```python
from build123d import *

# Parameters (mm, degrees)
F0_W     = 50.8
F0_H     = 33.02
F0_W_2   = 40.64
F0_H_2   = 22.86
F1_DEPTH = 17.78
F2_DEPTH = 12.7
F3_R     = 3.175
F4_DEPTH = 254


with BuildPart() as f1:
    # F0 (on Top) → F1 (new body)
    with BuildSketch(Plane.XY):
        with Locations((-7.5921734202, -29.6402639918)):
            Rectangle(F0_W, F0_H)
        with Locations((-7.5921734202, -29.6402639918)):
            Rectangle(F0_W_2, F0_H_2, mode=Mode.SUBTRACT)
        with Locations((-7.5921734202, -29.6402639918)):
            Rectangle(F0_W_2, F0_H_2)
    extrude(amount=F1_DEPTH)

    # F0 (on Top) → F2 (cut)
    with BuildSketch(Plane.XY):
        with Locations((-7.5921734202, -29.6402639918)):
            Rectangle(F0_W_2, F0_H_2)
    extrude(amount=F2_DEPTH, mode=Mode.SUBTRACT)

    # F3 (on face) → F4 (cut)
    with BuildSketch(Plane(origin=(-32.9921734202, 0, 0), x_dir=(0, -1, 0), z_dir=(-1, 0, 0))):
        with Locations((29.6402639918, 9.4274014091)):
            Circle(F3_R)
    extrude(amount=-F4_DEPTH, mode=Mode.SUBTRACT)


solid = f1.part
```
Can you work these out from the model? Positions are in its coordinate system, mm. A direction names the side the tool comes from. Coordinates: 2 decimals unless noted, no trailing zeros. Loops run counter-clockwise (first coordinate to the right, second up) from the corner with the lowest first, then second, coordinate; pieces in that order, holes last. Notation, with made-up numbers: (-23, -16) -> (-9, -16) arc R23 ccw to (-9, -6) -> close; hole circle Ø4 at (13, 75). An arc over 180 degrees is marked (long way). Answer as a JSON object with one key per item and string values.
1) Thinking about a two-plate mould opening in Y: for faces 1 (the face through (-27.912, -30, 5)), 2 (the face through (17.808, -26, 9)), 3 (the face through (-30.488, -32.573, 8.211)), 4 (the face through (-8, -46.15, 9)), which applies, pulls with the +Y half, pulls with the -Y half, needs draft (parallel to the pull), parting line crosses it, or undercut?
Results:
{"face 1": "undercut", "face 2": "needs draft", "face 3": "undercut", "face 4": "pulls with the -Y half"}
2) For P1, Ø1.5, axis at x = -6.5, y = -20.5, coming from the -Z side, with a flat end and sliding along its axis, tell me the tip position at first contact or that it passes through.
Results:
{"P1": "stops at z = 12.7"}
3) Imagine slicing it at B-B (x = -4). Please give me the cut outline in (y, z), then the cut area to 3 significant figures.
Results:
{"outline": "(-46.15, 0) -> (-41.07, 0) -> (-41.07, 12.7) -> (-18.21, 12.7) -> (-18.21, 0) -> (-13.13, 0) -> (-13.13, 17.78) -> (-46.15, 17.78) -> close", "area": "297 mm^2"}
4) Imagine slicing it at C-C (y = -34.5). Please give me the cut outline in (x, z).
Results:
{"outline": "(-32.99, 0) -> (-27.91, 0) -> (-27.91, 12.7) -> (12.73, 12.7) -> (12.73, 0) -> (17.81, 0) -> (17.81, 17.78) -> (-32.99, 17.78) -> close"}
5) Imagine slicing it at A-A (z = 2). Please give me the cut outline in (x, y).
Results:
{"outline": "(-32.99, -46.15) -> (17.81, -46.15) -> (17.81, -13.13) -> (-32.99, -13.13) -> close; hole (-27.91, -41.07) -> (12.73, -41.07) -> (12.73, -18.21) -> (-27.91, -18.21) -> close"}
6) If I drill on line 1 (Y direction, x = -17, z = 4.75); line 2 (X direction, y = -31.5, z = 2.25); line 3 (Z direction, x = -0.5, y = -27), over which ranges is the centre line in solid material (lowest first)?
Results:
{"line 1": "y = -46.15 to -41.07, -18.21 to -13.13", "line 2": "x = -32.99 to -27.91, 12.73 to 17.81", "line 3": "z = 12.7 to 17.78"}
7) Imagine slicing it at D-D (z = 8). Please give me the cut outline in (x, y).
Results:
{"outline": "(-32.99, -46.15) -> (17.81, -46.15) -> (17.81, -32.48) -> (12.73, -32.48) -> (12.73, -41.07) -> (-27.91, -41.07) -> (-27.91, -32.48) -> (-32.99, -32.48) -> close; (-32.99, -26.8) -> (-27.91, -26.8) -> (-27.91, -18.21) -> (12.73, -18.21) -> (12.73, -26.8) -> (17.81, -26.8) -> (17.81, -13.13) -> (-32.99, -13.13) -> close"}
8) For faces 5 (the face through (-8, -13.13, 9)), 6 (the face through (-8, -18.21, 6)), which set-ups out of +Z, -Z, +X, -X, +Y, -Y let a thin tool reach every point of the face, with its end or its side?
Results:
{"face 5": "+Z, -Z, +X, -X, +Y", "face 6": "-Z"}
